For this review, take the finished solid that the model builds, in its own axes (mm). Round coordinates to 2 decimals unless told otherwise and drop trailing zeros. Write each loop counter-clockwise with the first axis right and the second up, starting at its lowest first coordinate (ties: lowest second). Pieces come first, ordered by that corner, then holes. Notation, with made-up numbers: (87.25, -9.75) -> (91.25, -9.75) arc R25 ccw to (91.25, 27.25) -> close; hole circle Ø5 at (-26, 55). An arc over 180 degrees is marked (long way). Write each question's results on one line, items separated by ' | '. Start each with the question number.
Item 1: To check wall thickness, follow line 1 along Y through (x, z) = (-9.15, 0); line 2 along Y through (x, z) = (-11.5, -26); line 3 along Z through (x, y) = (-16.25, -24). State the ranges of each line that lie inside material, in increasing order.
Item 2: Add section D-D (x = -14.25). State the section outline as (y, z) points, plus the area to 3 significant figures.
Item 3: Add section A-A (y = 0). State the section outline as (x, z) points.
Item 4: Clearance check with flat-ended pins moving along their axes: pin 1 (8 mm diameter, centred on y = -22.5, z = 9, fed in from +X); pin 2 (10 mm diameter, centred on x = -15, z = -10, fed in from -Y); pin 3 (3 mm diameter, centred on x = -19.5, z = -8, fed in from -Y); pin 4 (6 mm diameter, centred on x = -15, y = 7, fed in from -Z). State where each tip first meets the part, or that it passes through.
Item 5: The part is to be moulded in two halves that separate along Z. For faces 1 (the flat face through (-24.488, 27, 16)), 2 (the cylindrical face through (-15.39, 33.44, 17.39)), 3 (the cylindrical face through (-8.439, -9.231, 29.314)), say which applies: +Z half, -Z half, draft (parallel to the pull), parting line (faces both ways), or undercut.
Item 6: Add section C-C (x = -19.75). State the section outline as (y, z) points, plus the area to 3 significant figures.
from build123d import *

# Parameters (mm, degrees)
FILLET1_R    = 2.1
SCALE1_SCALE = 0.2
SCALE2_SCALE = 1.9329
SCALE3_SCALE = 1.5


with BuildPart() as part:
    # Sketch1 → Revolve1 (revolve)
    with BuildSketch(Plane.XY, mode=Mode.PRIVATE) as revolve1_sk:
        with BuildLine():
            Line((-31, 65), (0, 65))
            Line((0, 65), (0, 53))
            Line((0, 53), (-6.55572809, 53))
            ThreePointArc((-6.55572809, 53), (-15.5, 57), (-24.44427191, 53))
            Line((-24.44427191, 53), (-31, 53))
            Line((-31, 53), (-31, 65))
        make_face()
    revolve(revolve1_sk.sketch.rotate(Axis((-28.722748815, 0, 0), (1, 0, 0)), 90), axis=Axis((-28.722748815, 0, 0), (1, 0, 0)))

    # Fillet1
    fillet1_edges = [part.edges().sort_by_distance(p)[0] for p in [
        (-31, 0, -65),
        (0, 0, -65),
    ]]
    fillet(fillet1_edges, radius=FILLET1_R)


with BuildPart() as part_1:
    # Scale1: scaled about (-15.5, 0, 0)
    add(part.part.scale(SCALE1_SCALE).moved(Location((-12.4, 0, 0))))


with BuildPart() as part_2:
    # Scale2: scaled about (-15.5, 0, 0)
    add(part_1.part.scale(SCALE2_SCALE).moved(Location((14.45995, 0, 0))))


with BuildPart() as part_3:
    # Scale3: scaled about (-15.5, 0, 0)
    add(part_2.part.scale(SCALE3_SCALE).moved(Location((7.75, 0, 0))))


solid = part_3.part
Responses:
1) line 1: y = -37.69 to -30.73, 30.73 to 37.69 | line 2: y = -27.29 to -18.29, 18.29 to 27.29 | line 3: z = -29.06 to -22.67, 22.67 to 29.06
2) outline: circle Ø75.38 at (0, 0); hole circle Ø65.88 at (0, 0) | area: 1,050 mm^2
3) outline: (-24.49, -36.47) arc R1.22 ccw to (-23.27, -37.69) -> (-7.73, -37.69) arc R1.22 ccw to (-6.51, -36.47) -> (-6.51, -30.73) -> (-10.31, -30.73) arc R6.96 cw to (-20.69, -30.73) -> (-24.49, -30.73) -> close; (-24.49, 30.73) -> (-20.69, 30.73) arc R6.96 cw to (-10.31, 30.73) -> (-6.51, 30.73) -> (-6.51, 36.47) arc R1.22 ccw to (-7.73, 37.69) -> (-23.27, 37.69) arc R1.22 ccw to (-24.49, 36.47) -> close
4) pin 1: passes through | pin 2: stops at y = -37.36 | pin 3: stops at y = -37.13 | pin 4: stops at z = -37.48
5) face 1: draft | face 2: parting line | face 3: undercut
6) outline: circle Ø75.38 at (0, 0); hole circle Ø63.21 at (0, 0) | area: 1,330 mm^2
